Autodesk Inventor part; units mm, degrees
ref_plane "YZ Plane" through (0, 0, 0) normal (1, 0, 0) x (0, 1, 0)
ref_plane "XZ Plane" through (0, 0, 0) normal (0, 1, 0) x (-1, 0, 0)
ref_plane "XY Plane" through (0, 0, 0) normal (0, 0, 1) x (1, 0, 0)
sketch "Sketch1" plane through (0, 0, 0) normal (0, 1, 0) x (-1, 0, 0)
  line L0 (-5, 20) -> (-5, 8)
  line L1 (5, -20) -> (5, -8)
  line L2 (20, 5) -> (8, 5)
  line L3 (-20, -5) -> (-8, -5)
  line L4 (8, -5) -> (20, -5)
  line L5 (-8, 5) -> (-20, 5)
  line L6 (-5, -8) -> (-5, -20)
  line L7 (5, 8) -> (5, 20)
  arc A0 (-17, 20) -> (-20, 17) centre (-17, 17) ccw
  arc A1 (-20, -17) -> (-17, -20) centre (-17, -17) ccw
  arc A2 (17, -20) -> (20, -17) centre (17, -17) ccw
  arc A3 (20, 17) -> (17, 20) centre (17, 17) ccw
  line L8 (20, 17) -> (20, 5)
  line L9 (20, -5) -> (20, -17)
  line L10 (17, -20) -> (5, -20)
  line L11 (-5, -20) -> (-17, -20)
  line L12 (-20, -17) -> (-20, -5)
  line L13 (-20, 5) -> (-20, 17)
  line L14 (-17, 20) -> (-5, 20)
  line L15 (17, 20) -> (5, 20)
  line L16 (5, 8) -> (-5, 8)
  line L17 (-8, 5) -> (-8, -5)
  line L18 (-5, -8) -> (5, -8)
  line L19 (8, -5) -> (8, 5)
  point P0 (0, 0)
extrude "Extrusion1" add sketch "Sketch1" along normal blind 1200
properties part number "column"
Geometry: final body of the model. Coordinates: model frame, mm. Round coordinates to 2 decimals unless told otherwise and drop trailing zeros. Write each loop counter-clockwise with the first axis right and the second up, starting at its lowest first coordinate (ties: lowest second). Pieces come first, ordered by that corner, then holes.
Item 1: Pin query (flat end, axial travel): P1, Ø8, axis at y = 505, z = -0.5, coming from the -X side; P2, Ø8, axis at y = 537.5, z = 0, coming from the +X side; P3, Ø6, axis at x = 1, y = 895.5, coming from the -Z side. Return the tip coordinate at first contact, or that it passes through.
Item 2: Section query A-A (y = 1022.5). Return loops of the section in (x, z).
Item 3: Material intervals for L1, parallel to X at y = 1147.5, z = -9.5; L2, parallel to X at y = 808.5, z = 1, sorted ascending.
Completed:
1. P1: stops at x = -8
1. P2: stops at x = 8
1. P3: stops at z = -8
2. outline: (-20, -17) arc R3 ccw to (-17, -20) - (-5, -20) - (-5, -8) - (5, -8) - (5, -20) - (17, -20) arc R3 ccw to (20, -17) - (20, -5) - (8, -5) - (8, 5) - (20, 5) - (20, 17) arc R3 ccw to (17, 20) - (5, 20) - (5, 8) - (-5, 8) - (-5, 20) - (-17, 20) arc R3 ccw to (-20, 17) - (-20, 5) - (-8, 5) - (-8, -5) - (-20, -5) - close
3. L1: x = -20 to -5, 5 to 20
3. L2: x = -8 to 8
